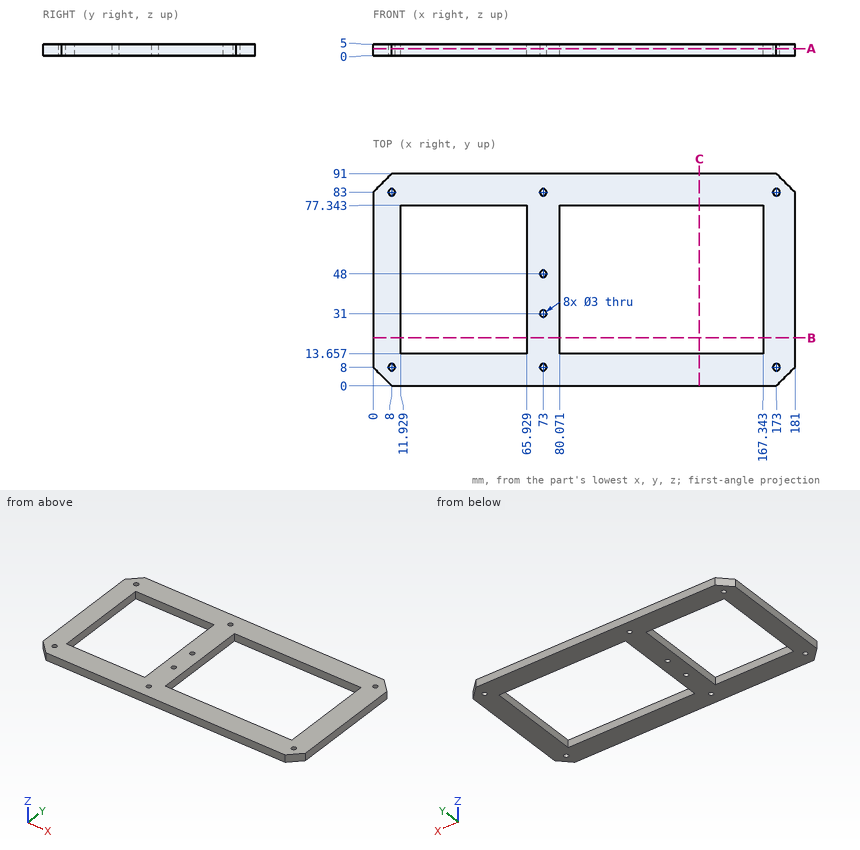
The figure shows three views and two pictorial views of one solid part (mm, origin at its lowest corner). Answer the questions. Give positions to 0.01 mm unless a question says otherwise; leave off trailing zeros. Order: outer loops, then holes, each group sorted by start corner. A loop starts at its lowest first (then second) coordinate and runs counter-clockwise, first axis right, second up. Notation, with made-up numbers: (28.25, 67) -> (40.25, 67) arc R10 ccw to (40.25, 86) -> close; hole circle Ø3 at (81, -10). An arc over 180 degrees is marked (long way). Answer as CSV lines item,"result". Start each with the question number.
Q1. A cutting plane is placed at A-A (z = 3). Count the separate pieces of the cut face and the enclosed holes in it, then the cut area to 3 significant figures.
Q2. Find the intervals of material crossed by L1, parallel to X at y = 68, z = 1.2; L2, parallel to Y at x = 131, z = 2.1; L3, parallel to Y at x = 8.5, z = 0.7, in increasing order.
Q3. A cutting plane is placed at C-C (x = 140). Determine the outline of the cut face in (y, z).
Q4. Given pin 1 (2.5 mm diameter, centred on x = 73, y = 48, fed in from -Z), flat-ended and moving along its own axis, determine where the tip first touches the part or whether it passes through.
Q5. A cutting plane is placed at B-B (y = 20.5). Determine the outline of the cut face in (x, z).
Results found:
1,separate pieces,"1"
1,enclosed holes,"10"
1,area,"7,290 mm2"
2,L1,"0 to 11.93, 65.93 to 80.07, 167.34 to 181"
2,L2,"0 to 13.66, 77.34 to 91"
2,L3,"0 to 6.59, 9.41 to 81.59, 84.41 to 91"
3,outline,"(0, 0) -> (13.66, 0) -> (13.66, 5) -> (0, 5) -> close; (77.34, 0) -> (91, 0) -> (91, 5) -> (77.34, 5) -> close"
4,pin 1,"through"
5,outline,"(0, 0) -> (11.93, 0) -> (11.93, 5) -> (0, 5) -> close; (65.93, 0) -> (80.07, 0) -> (80.07, 5) -> (65.93, 5) -> close; (167.34, 0) -> (181, 0) -> (181, 5) -> (167.34, 5) -> close"
